```python
from build123d import *

# Parameters (mm, degrees)
BOSS_EXTRUDE6_DEPTH            = 500
M5_CLEARANCE_HOLE1_D           = 5.5
M5_CLEARANCE_HOLE1_CSINK_D     = 5.55
M5_CLEARANCE_HOLE1_CSINK_ANGLE = 90


with BuildPart() as part:
    # Sketch4 → Boss-Extrude6 (new body)
    with BuildSketch(Plane.XY):
        Polygon((0, 0), (50, 0), (67.101007166, -46.984631039), (63.887069118, -48.154408824), (50, -10), (0, -10), align=None)
    extrude(amount=BOSS_EXTRUDE6_DEPTH)

    # M5 Clearance Hole1 (through all)
    with Locations(Plane(origin=(44.151111078, 16.069690242, 0), x_dir=(0, 0, -1), z_dir=(0.939692621, 0.342020143, 0))):
        with Locations((-325, -37.141900038), (-325, -62.141900038), (-175, -62.141900038), (-175, -37.141900038)):
            CounterSinkHole(M5_CLEARANCE_HOLE1_D / 2, M5_CLEARANCE_HOLE1_CSINK_D / 2, counter_sink_angle=M5_CLEARANCE_HOLE1_CSINK_ANGLE)


solid = part.part
```
The listing builds one solid part. Answer for the finished solid, in the listing's coordinates (mm). A direction names the side the tool comes from. Coordinates: 2 decimals unless noted, no trailing zeros. Loops run counter-clockwise (first coordinate to the right, second up) from the corner with the lowest first, then second, coordinate; pieces in that order, holes last. Notation, with made-up numbers: (29.25, 31.5) -> (87.25, 31.5) arc R22 ccw to (87.25, 66.5) -> close; hole circle Ø9 at (42.5, 48.25). An arc over 180 degrees is marked (long way). Return JSON: item names as keys, results as strings. Group by question number.
(1) Given pin 1 Ø1 at (y, z) = (-22, 299.5) entering from +X; pin 2 Ø10 at (y, z) = (-22, 358.5) entering from -X; pin 3 Ø5 at (y, z) = (-41.5, 239.5) entering from -X, each flat-ended and moving along its own axis, determine where each tip first touches the part or whether it passes through.
(2) Find the intervals of material crossed by probe 1 along Y at (x, z) = (5.5, 109.5); probe 2 along X at (y, z) = (-11, 204); probe 3 along X at (y, z) = (-15, 140), in increasing order. Write a range as from..to.
(3) A cutting plane is placed at B-B on x = 22. Write down the section's boundary in (y, z), and give its area (3 significant figures).
(4) A cutting plane is placed at C-C on y = -5. Write down the section's boundary in (x, z).
(5) A cutting plane is placed at A-A on z = 283. Write down the section's boundary in (x, y).
(6) Which of the six approach directions +Z, -Z, +X, -X, +Y, -Y give full straight-line access (tool end or side, diameter ignored) to faces 1 (the flat face through (0, -5, 246)), 2 (the flat face through (25, -10, 246))?
The answers:
{
 "1": {"pin 1": "stops at x = 58.19", "pin 2": "stops at x = 52.55", "pin 3": "stops at x = 60.56"},
 "2": {"probe 1": "y = -10..0", "probe 2": "x = 50.36..54", "probe 3": "x = 51.82..55.46"},
 "3": {"outline": "(-10, 0) -> (0, 0) -> (0, 500) -> (-10, 500) -> close", "area": "5,000 mm^2"},
 "4": {"outline": "(0, 0) -> (51.82, 0) -> (51.82, 500) -> (0, 500) -> close"},
 "5": {"outline": "(0, -10) -> (50, -10) -> (63.89, -48.15) -> (67.1, -46.98) -> (50, 0) -> (0, 0) -> close"},
 "6": {"face 1": "+Z, -Z, -X, +Y, -Y", "face 2": "+Z, -Z, -X, -Y"}
}
